Geometry check sheet. Reference: the model listing, model coordinates, mm. A direction names the side the tool comes from. Round coordinates to 2 decimals unless told otherwise and drop trailing zeros. Write each loop counter-clockwise with the first axis right and the second up, starting at its lowest first coordinate (ties: lowest second). Pieces come first, ordered by that corner, then holes.
Item 1: Cross-section at B-B (y = 0). State how many separate pieces and enclosed holes the cut face has, then the cut area to 3 significant figures.
Item 2: Draft check along Z on faces 1 (the face through (27.878, -18, -27)), 2 (the face through (0.42, -13.07, -58.87)), 3 (the face through (32, 0, 0)). Enter one of: pulls with the +Z half, pulls with the -Z half, needs draft (parallel to the pull), parting line crosses it, or undercut.
Item 3: Access from +Z, -Z, +X, -X, +Y, -Y to the whole of each face (thin tool, end or side, straight path). Record for faces 4 (the face through (-27.878, 18, -27)), 5 (the face through (30.385, 27.712, -11.49)), 6 (the face through (-30.782, -21, 22)), 7 (the face through (-60, 0, 0)).
Item 4: Depth check by flat-ended pin: P1, Ø1, axis at x = 30.5, y = -16.5, coming from the +Z side; P2, Ø10, axis at y = 40, z = -37, coming from the -X side; P3, Ø8, axis at y = 41, z = -3, coming from the -X side. Enter the tip coordinate at first touch or a pass-through.
Item 5: Scan lines: probe 1 along Z at (x, y) = (14, 0); probe 2 along X at (y, z) = (11, -34.5); probe 3 along Y at (x, z) = (10.5, 3.5). Record each from-to range of solid material in increasing order.
Item 6: Cross-section at A-A (x = -8). Enter the section's corners in (y, z).
from build123d import *

# Parameters (mm, degrees)
REVOLVE_1_OUTLINE_W   = 0.355269541
REVOLVE_1_OUTLINE_H   = 0.438478825
REVOLVE_1_OUTLINE_W_2 = 11.364624133
REVOLVE_1_OUTLINE_W_3 = 4.372569082
REVOLVE_1_OUTLINE_H_2 = 55.75634902
REVOLVE_1_OUTLINE_H_3 = 1.854936884
REVOLVE_1_OUTLINE_W_4 = 14.211965544
REVOLVE_1_OUTLINE_H_4 = 0.61022171
SKETCH_2_R            = 30
EXTRUDE_1_DEPTH       = 30
SKETCH_3_R            = 8
EXTRUDE_2_DEPTH       = 30
SKETCH_4_W            = 5
SKETCH_4_H            = 22.5
SKETCH_4_W_2          = 22.5
SKETCH_4_H_2          = 5
EXTRUDE_3_DEPTH       = 2


# Read off the part's stored shape, not the designer's step: 회전1
with BuildPart() as part:
    # 회전1 outline → 회전1 (revolve)
    with BuildSketch(Plane.YX):
        with Locations((41.542258903, -28.097413923)):
            Rectangle(REVOLVE_1_OUTLINE_W, REVOLVE_1_OUTLINE_H)
        with BuildLine():
            add(Edge.make_bspline(
                [(41.719893674, -27.87817451), (41.894749248, -27.921618592), (42.252720208, -28.01137838), (42.873298399, -28.15700866), (43.341279515, -28.256769587), (43.642191366, -28.316653335)],
                knots=[0.117139278, 0.117139278, 0.117139278, 0.117139278, 0.14529069, 0.173442101, 0.224513922, 0.224513922, 0.224513922, 0.224513922], degree=3))
            Line((41.719893674, -27.87817451), (41.719893674, -28.316653335))
            Line((41.719893674, -28.316653335), (43.642191366, -28.316653335))
        make_face()
        with BuildLine():
            add(Edge.make_bspline(
                [(43.642191366, -28.316653335), (43.673012094, -28.322786894), (44.367114713, -28.459908676), (46.367881136, -28.788520691), (49.637320271, -29.015805628), (53.021708434, -28.821695589), (55.131271584, -28.478533008), (55.931859218, -28.316653335)],
                knots=[0.224513922, 0.224513922, 0.224513922, 0.224513922, 0.229744924, 0.34235057, 0.567561862, 0.792773154, 0.932194296, 0.932194296, 0.932194296, 0.932194296], degree=3))
            Line((43.642191366, -28.316653335), (41.719893674, -28.316653335))
            Line((41.719893674, -28.316653335), (41.719893674, -30.171590219))
            Line((41.719893674, -30.171590219), (55.931859218, -30.171590219))
            Line((55.931859218, -30.171590219), (55.931859218, -28.316653335))
        make_face()
        with Locations((35.682312067, -28.097413923)):
            Rectangle(REVOLVE_1_OUTLINE_W_2, REVOLVE_1_OUTLINE_H)
        with Locations((58.118143759, -28.097413923)):
            Rectangle(REVOLVE_1_OUTLINE_W_3, REVOLVE_1_OUTLINE_H)
        with Locations((58.118143759, 0)):
            Rectangle(REVOLVE_1_OUTLINE_W_3, REVOLVE_1_OUTLINE_H_2)
        with BuildLine():
            Line((41.719893674, 28.316653335), (41.719893674, 27.87817451))
            add(Edge.make_bspline(
                [(43.128876316, 28.316653335), (42.973861456, 28.272694047), (42.669494175, 28.183372992), (42.227403007, 28.044794313), (41.884836208, 27.931979132), (41.719893674, 27.87817451)],
                knots=[0.937972384, 0.937972384, 0.937972384, 0.937972384, 0.966974102, 0.995182728, 1.023391355, 1.023391355, 1.023391355, 1.023391355], degree=3))
            Line((43.128876316, 28.316653335), (41.719893674, 28.316653335))
        make_face()
        with Locations((41.542258903, 28.097413923)):
            Rectangle(REVOLVE_1_OUTLINE_W, REVOLVE_1_OUTLINE_H)
        with Locations((41.542258903, -29.244121777)):
            Rectangle(REVOLVE_1_OUTLINE_W, REVOLVE_1_OUTLINE_H_3)
        with Locations((58.118143759, -29.244121777)):
            Rectangle(REVOLVE_1_OUTLINE_W_3, REVOLVE_1_OUTLINE_H_3)
        with Locations((35.682312067, -29.244121777)):
            Rectangle(REVOLVE_1_OUTLINE_W_2, REVOLVE_1_OUTLINE_H_3)
        with Locations((35.682312067, 28.097413923)):
            Rectangle(REVOLVE_1_OUTLINE_W_2, REVOLVE_1_OUTLINE_H)
        with Locations((58.118143759, 28.097413923)):
            Rectangle(REVOLVE_1_OUTLINE_W_3, REVOLVE_1_OUTLINE_H)
        with BuildLine():
            Line((41.719893674, 28.316653335), (43.128876316, 28.316653335))
            add(Edge.make_bspline(
                [(55.931859218, 28.316653335), (55.350466054, 28.484554725), (54.483083768, 28.700477141), (53.332821917, 28.919070087), (52.621816991, 29.026887301), (51.140275095, 29.207221888), (48.779721438, 29.304602769), (45.95584246, 28.998713875), (44.028351242, 28.564756145), (43.275412999, 28.358208372), (43.128876316, 28.316653335)],
                knots=[0.120715306, 0.120715306, 0.120715306, 0.120715306, 0.233549812, 0.285972839, 0.342390092, 0.370598718, 0.57205333, 0.797722342, 0.910556849, 0.937972384, 0.937972384, 0.937972384, 0.937972384], degree=3))
            Line((55.931859218, 28.316653335), (55.931859218, 30.171590219))
            Line((55.931859218, 30.171590219), (41.719893674, 30.171590219))
            Line((41.719893674, 30.171590219), (41.719893674, 28.316653335))
        make_face()
        with Locations((41.542258903, 29.244121777)):
            Rectangle(REVOLVE_1_OUTLINE_W, REVOLVE_1_OUTLINE_H_3)
        with Locations((48.825876446, -30.476701074)):
            Rectangle(REVOLVE_1_OUTLINE_W_4, REVOLVE_1_OUTLINE_H_4)
        with Locations((41.542258903, -30.476701074)):
            Rectangle(REVOLVE_1_OUTLINE_W, REVOLVE_1_OUTLINE_H_4)
        with BuildLine():
            Line((60.3044283, -30.171590219), (55.931859218, -30.171590219))
            Line((55.931859218, -30.171590219), (55.931859218, -30.781811929))
            Line((55.931859218, -30.781811929), (58.176696805, -30.781811929))
            add(Edge.make_bspline(
                [(60.3044283, -30.171590219), (59.242057092, -30.511353598), (58.176696805, -30.781811929)],
                knots=[0, 0, 0, 0.113573553, 0.113573553, 0.113573553], degree=2))
        make_face()
        with Locations((35.682312067, -30.476701074)):
            Rectangle(REVOLVE_1_OUTLINE_W_2, REVOLVE_1_OUTLINE_H_4)
        with Locations((35.682312067, 29.244121777)):
            Rectangle(REVOLVE_1_OUTLINE_W_2, REVOLVE_1_OUTLINE_H_3)
        with Locations((58.118143759, 29.244121777)):
            Rectangle(REVOLVE_1_OUTLINE_W_3, REVOLVE_1_OUTLINE_H_3)
        with Locations((41.542258903, 30.476701074)):
            Rectangle(REVOLVE_1_OUTLINE_W, REVOLVE_1_OUTLINE_H_4)
        with Locations((48.825876446, 30.476701074)):
            Rectangle(REVOLVE_1_OUTLINE_W_4, REVOLVE_1_OUTLINE_H_4)
        with BuildLine():
            Line((55.931859218, -30.781811929), (41.719893674, -30.781811929))
            Line((41.719893674, -30.781811929), (41.719893674, -30.868243844))
            add(Edge.make_bspline(
                [(49.816181075, -31.837257545), (45.788933817, -31.837257541), (41.719893674, -30.868243844)],
                knots=[0.556786778, 0.556786778, 0.556786778, 0.981464752, 0.981464752, 0.981464752], degree=2))
            add(Edge.make_bspline(
                [(55.931859218, -31.274158213), (52.886163188, -31.837257547), (49.816181075, -31.837257545)],
                knots=[0.233053543, 0.233053543, 0.233053543, 0.556786778, 0.556786778, 0.556786778], degree=2))
            Line((55.931859218, -31.274158213), (55.931859218, -30.781811929))
        make_face()
        with BuildLine():
            Line((41.719893674, -30.868243844), (41.719893674, -30.781811929))
            Line((41.719893674, -30.781811929), (41.364624133, -30.781811929))
            add(Edge.make_bspline(
                [(41.719893674, -30.868243844), (41.54229871, -30.825950834), (41.364624133, -30.781811929)],
                knots=[0.981464752, 0.981464752, 0.981464752, 1, 1, 1], degree=2))
        make_face()
        with BuildLine():
            Line((58.176696805, -30.781811929), (55.931859218, -30.781811929))
            Line((55.931859218, -30.781811929), (55.931859218, -31.274158213))
            add(Edge.make_bspline(
                [(58.176696805, -30.781811929), (57.055932041, -31.066335551), (55.931859218, -31.274158213)],
                knots=[0.113573553, 0.113573553, 0.113573553, 0.233053543, 0.233053543, 0.233053543], degree=2))
        make_face()
        with Locations((35.682312067, 30.476701074)):
            Rectangle(REVOLVE_1_OUTLINE_W_2, REVOLVE_1_OUTLINE_H_4)
        with BuildLine():
            Line((55.931859218, 30.781811929), (55.931859218, 30.171590219))
            Line((55.931859218, 30.171590219), (60.3044283, 30.171590219))
            add(Edge.make_bspline(
                [(58.176696805, 30.781811929), (59.242057092, 30.511353598), (60.3044283, 30.171590219)],
                knots=[0.886426447, 0.886426447, 0.886426447, 1, 1, 1], degree=2))
            Line((58.176696805, 30.781811929), (55.931859218, 30.781811929))
        make_face()
        with BuildLine():
            Line((41.364624133, 30.781811929), (41.719893674, 30.781811929))
            Line((41.719893674, 30.781811929), (41.719893674, 30.868243844))
            add(Edge.make_bspline(
                [(41.364624133, 30.781811929), (41.54229871, 30.825950834), (41.719893674, 30.868243844)],
                knots=[0, 0, 0, 0.018535248, 0.018535248, 0.018535248], degree=2))
        make_face()
        with BuildLine():
            Line((41.719893674, 30.868243844), (41.719893674, 30.781811929))
            Line((41.719893674, 30.781811929), (55.931859218, 30.781811929))
            Line((55.931859218, 30.781811929), (55.931859218, 31.274158213))
            add(Edge.make_bspline(
                [(49.816181262, 31.837257545), (52.886163281, 31.83725753), (55.931859218, 31.274158213)],
                knots=[0.443213232, 0.443213232, 0.443213232, 0.766946457, 0.766946457, 0.766946457], degree=2))
            add(Edge.make_bspline(
                [(41.719893674, 30.868243844), (45.788933912, 31.837257564), (49.816181262, 31.837257545)],
                knots=[0.018535248, 0.018535248, 0.018535248, 0.443213232, 0.443213232, 0.443213232], degree=2))
        make_face()
        with BuildLine():
            Line((55.931859218, 31.274158213), (55.931859218, 30.781811929))
            Line((55.931859218, 30.781811929), (58.176696805, 30.781811929))
            add(Edge.make_bspline(
                [(55.931859218, 31.274158213), (57.055932041, 31.066335551), (58.176696805, 30.781811929)],
                knots=[0.766946457, 0.766946457, 0.766946457, 0.886426447, 0.886426447, 0.886426447], degree=2))
        make_face()
    revolve(axis=Axis((0, 0, 0), (1, 0, 0)))

    # 스케치2 → 보스-돌출1 (add, symmetric)
    with BuildSketch(Plane(origin=(0, 0, 0), x_dir=(0, 0, -1), z_dir=(1, 0, 0))):
        with Locations(Location((0, 0, 0), (0, 0, 270))):
            Circle(SKETCH_2_R)
    extrude(amount=EXTRUDE_1_DEPTH, both=True)

    # 스케치3 → 보스-돌출2 (add)
    with BuildSketch(Plane.ZY.offset(30)):
        with Locations(Location((0, 0, 0), (0, 0, 180))):
            Circle(SKETCH_3_R)
    extrude(amount=EXTRUDE_2_DEPTH)

    # 스케치4 → 보스-돌출3 (add)
    with BuildSketch(Plane(origin=(30, 0, 0), x_dir=(0, 0, -1), z_dir=(1, 0, 0))):
        with Locations((0, 13.75)):
            Rectangle(SKETCH_4_W, SKETCH_4_H)
        with Locations((-13.75, 0)):
            Rectangle(SKETCH_4_W_2, SKETCH_4_H_2)
        Rectangle(SKETCH_4_W, SKETCH_4_H_2)
        with Locations((13.75, 0)):
            Rectangle(SKETCH_4_W_2, SKETCH_4_H_2)
        with Locations((0, -13.75)):
            Rectangle(SKETCH_4_W, SKETCH_4_H)
    extrude(amount=EXTRUDE_3_DEPTH)


solid = part.part
Resolved:
1. separate pieces: 1
1. enclosed holes: 2
1. area: 5,020 mm2
2. face 1: undercut
2. face 2: parting line crosses it
2. face 3: needs draft
3. face 4: none
3. face 5: +X
3. face 6: -X
3. face 7: +Z, -Z, -X, +Y, -Y
4. P1: stops at z = 58.11
4. P2: stops at x = -31.84
4. P3: stops at x = -31.51
5. probe 1: z = -60.3 to -55.93, -30 to 30, 55.93 to 60.3
5. probe 2: x = -30.78 to -27.88, 27.88 to 30.78
5. probe 3: y = -60.2 to -55.82, -29.8 to 29.8, 55.82 to 60.2
6. outline: circle Ø120.61 at (0, 0); circle Ø60 at (0, 0); hole circle Ø111.86 at (0, 0)
